Can you work these out from the model? Positions are in its coordinate system, mm. Face numbers are marked on the shaded views. Give positions to 0.01 mm unless a question says otherwise; leave off trailing zeros. Loops run counter-clockwise (first coordinate to the right, second up) from the corner with the lowest first, then second, coordinate; pieces in that order, holes last. Notation, with made-up numbers: (-17.5, 67) - (24.5, 67) arc R15 cw to (24.5, 73) - close; hole circle Ø11 at (89, 3). An arc over 180 degrees is marked (long way). Use a Markdown table: item, result. Add a question column.
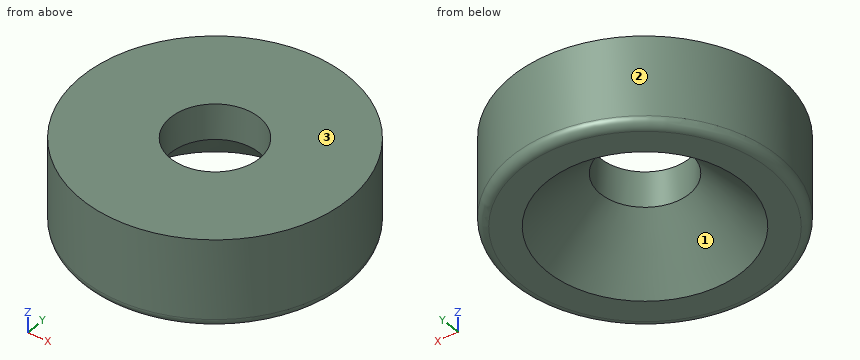
```python
from build123d import *

# Parameters (mm, degrees)
SKETCH_1_R      = 3
SKETCH_1_R_2    = 1
EXTRUDE_1_DEPTH = 2
CHAMFER_1_SIZE  = 1.2
FILLET_1_R      = 0.2


with BuildPart() as part:
    # 草图1 → 凸台-拉伸1 (new body)
    with BuildSketch(Plane.XY):
        Circle(SKETCH_1_R)
        Circle(SKETCH_1_R_2, mode=Mode.SUBTRACT)
    extrude(amount=EXTRUDE_1_DEPTH)

    # 倒角1
    chamfer_1_edges = [part.edges().sort_by_distance(p)[0] for p in [
        (-1, 0, 0),
    ]]
    chamfer(chamfer_1_edges, length=CHAMFER_1_SIZE)

    # 圆角1
    fillet_1_edges = [part.edges().sort_by_distance(p)[0] for p in [
        (-3, 0, 0),
    ]]
    fillet(fillet_1_edges, radius=FILLET_1_R)


solid = part.part
```
1. Please list where these lines run through material, in increasing order: line 1 along Y through (x, z) = (0, 1.85); line 2 along Y through (x, z) = (-0.5, 0.55); line 3 along X through (y, z) = (-0.5, 1.85). Write a range as [from, to].
2. Suppose I cut it at A-A (y = 0). List the corners of the cut face in (x, z) for me, and give its area (3 significant figures).
3. Suppose I cut it at C-C (z = 1.1). List the corners of the cut face in (x, y) for me.
4. If we mould it in two halves opening along Y, with no side actions, what happens to the marked faces 1, 2 and 3? For each: released by +Y, released by -Y, zero draft, split by the parting line, or undercut.
5. Suppose I cut it at D-D (z = 1.55). List the corners of the cut face in (x, y) for me, and give its area (3 significant figures).
Results below:
| question | item | result |
|---|---|---|
| 1 | line 1 | [-3, -1], [1, 3] |
| 1 | line 2 | [-2.96, -1.57], [1.57, 2.96] |
| 1 | line 3 | [-2.96, -0.87], [0.87, 2.96] |
| 2 | outline | (-3, 0.2) arc R0.2 ccw to (-2.8, 0) - (-2.2, 0) - (-1, 1.2) - (-1, 2) - (-3, 2) - close; (1, 1.2) - (2.2, 0) - (2.8, 0) arc R0.2 ccw to (3, 0.2) - (3, 2) - (1, 2) - close |
| 2 | area | 6.54 mm² |
| 3 | outline | circle Ø6 at (0, 0); hole circle Ø2.2 at (0, 0) |
| 4 | face 1 | undercut |
| 4 | face 2 | split by the parting line |
| 4 | face 3 | zero draft |
| 5 | outline | circle Ø6 at (0, 0); hole circle Ø2 at (0, 0) |
| 5 | area | 25.1 mm² |
